Can you work these out from the model? Positions are in its coordinate system, mm. Round coordinates to 2 decimals unless told otherwise and drop trailing zeros. Write each loop counter-clockwise with the first axis right and the second up, starting at its lowest first coordinate (ties: lowest second). Pieces come first, ordered by that corner, then holes. Notation, with made-up numbers: (61, 46.25) -> (77, 46.25) arc R20 cw to (77, 58.25) -> close; hole circle Ø2 at (-5.75, -18.75). An arc over 180 degrees is marked (long way). Write item = value, one per line. Start each with the question number.
1) Imagine slicing it at B-B, the plane z = 3. Please give me the cut outline in (x, y), then the cut area to 3 significant figures.
2) I'm going to push flat-ended pins straight in: pin 1 (8 mm diameter, centred on y = 57.5, z = -11.5, fed in from +X); pin 2 (2 mm diameter, centred on y = -50, z = 2, fed in from +X); pin 3 (4 mm diameter, centred on y = 52.5, z = -6, fed in from -X); pin 4 (9.5 mm diameter, centred on x = -1448.06, y = 75, fed in from +Z). Where does each tip first touch, or does it pass through?
3) If I drill on line 1 (Z direction, x = -1444.5, y = -43); line 2 (Z direction, x = -1450.5, y = -117); line 3 (X direction, y = -33, z = -3.5), over which ranges is the centre line in solid material (lowest first)?
4) Imagine slicing it at A-A, the plane z = -7.5. Please give me the cut outline in (x, y) (1 decimal).
from build123d import *
from build123d import SkipClean  # not in build123d's __all__

# Parameters (mm, degrees)
F0_R          = 15
F0_R_2        = 12
F1_ANGLE_BACK = 5
F1_ANGLE      = 10
F2_R          = 5.25
F3_DEPTH      = 15.001
F3_DEPTH_BACK = 15.001


with BuildPart() as f1:
    # F0 (on Front) → F1 (revolve)
    with BuildSketch(Plane.XZ, mode=Mode.PRIVATE) as f1_sk:
        with Locations((-1450, 0)):
            Circle(F0_R)
        with Locations((-1450, 0)):
            Circle(F0_R_2, mode=Mode.SUBTRACT)
    revolve(f1_sk.sketch.rotate(Axis((0, 0, 190.0846064091), (0, 0, -1)), -F1_ANGLE_BACK), axis=Axis((0, 0, 190.0846064091), (0, 0, -1)), revolution_arc=F1_ANGLE)

    # F2 (on Top) → F3 (cut, two sides)
    with BuildSketch(Plane.XY) as f3_sk:
        with Locations((-1448.0590457575, -75)):
            Circle(F2_R)
        with Locations((-1448.0590457575, 75)):
            Circle(F2_R)
    with SkipClean():  # cleaning this boolean's faces spoils the solid; the shape is the same uncleaned
        extrude(amount=-F3_DEPTH, mode=Mode.SUBTRACT)
        extrude(f3_sk.sketch, amount=F3_DEPTH_BACK, mode=Mode.SUBTRACT)


solid = f1.part
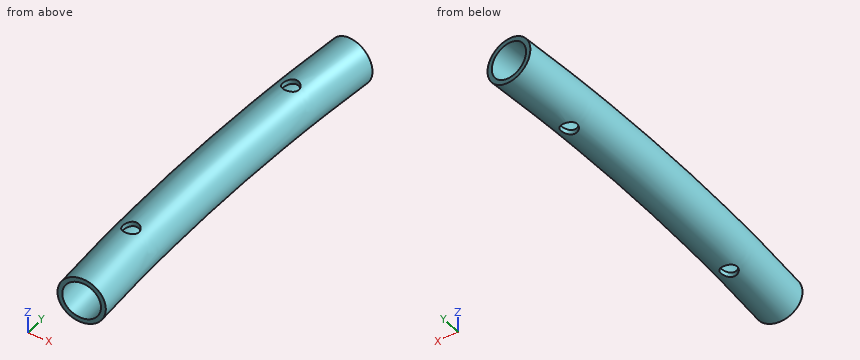
Reported:
q1.outline = (-1459.12, -127.66) -> (-1456.06, -127.39) arc R1461.62 cw to (-1456.06, 127.39) -> (-1459.12, 127.66) arc R1464.7 ccw to start; (-1432.91, -125.36) -> (-1429.84, -125.09) arc R1435.3 cw to (-1429.84, 125.09) -> (-1432.91, 125.36) arc R1438.38 ccw to start
q1.area = 1,560 mm²
q2.pin_1 = -1435.85
q2.pin_2 = -1434.15
q2.pin_3 = -1463.52
q2.pin_4 = through
q3.line_1 = -14.19 to -10.97, 10.97 to 14.19
q3.line_2 = -14.07 to -10.81, 10.81 to 14.07
q3.line_3 = -1464.21 to -1461.11, -1438.14 to -1435.03
q4.outline = (-1457.4, -127.5) -> (-1453.8, -127.2) arc R1459.4 cw to (-1453.8, 127.2) -> (-1457.4, 127.5) arc R1463 ccw to start; (-1435.2, -125.6) -> (-1431.5, -125.2) arc R1437 cw to (-1431.5, 125.2) -> (-1435.2, 125.6) arc R1440.6 ccw to start
